```python
from build123d import *

# Parameters (mm, degrees)
F0_R     = 1.524
F1_DEPTH = 38.1
F2_R     = 25.4
F3_DEPTH = 38.101


with BuildPart() as f1:
    # F0 (on Top) → F1 (new body)
    with BuildSketch(Plane.XY):
        with BuildLine():
            ThreePointArc((30.1625, 25.4), (28.767596, 28.767596), (25.4, 30.1625))
            Line((25.4, 30.1625), (-25.4, 30.1625))
            ThreePointArc((-25.4, 30.1625), (-28.767596, 28.767596), (-30.1625, 25.4))
            Line((-30.1625, 25.4), (-30.1625, -25.4))
            ThreePointArc((-30.1625, -25.4), (-28.767596, -28.767596), (-25.4, -30.1625))
            Line((-25.4, -30.1625), (25.4, -30.1625))
            ThreePointArc((25.4, -30.1625), (28.767596, -28.767596), (30.1625, -25.4))
            Line((30.1625, -25.4), (30.1625, 25.4))
        make_face()
        with Locations((-25.4, -25.4)):
            Circle(F0_R, mode=Mode.SUBTRACT)
        with Locations((25.4, -25.4)):
            Circle(F0_R, mode=Mode.SUBTRACT)
        with Locations((-25.4, 25.4)):
            Circle(F0_R, mode=Mode.SUBTRACT)
        with Locations((25.4, 25.4)):
            Circle(F0_R, mode=Mode.SUBTRACT)
    extrude(amount=F1_DEPTH)

    # F2 (on face) → F3 (cut, through all)
    with BuildSketch(Plane.XY.offset(38.1)):
        Circle(F2_R)
    extrude(amount=-F3_DEPTH, mode=Mode.SUBTRACT)


solid = f1.part
```
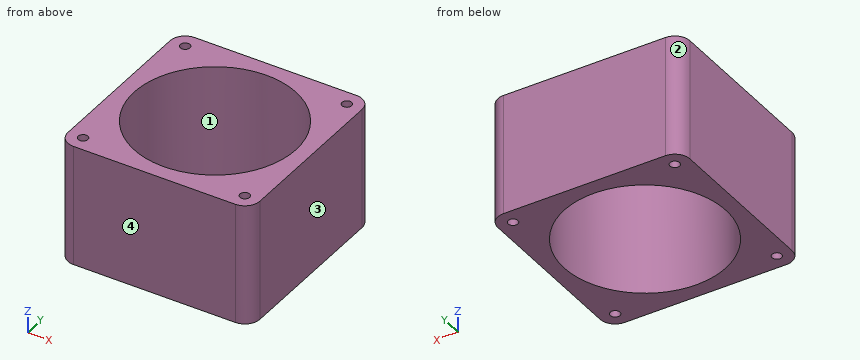
Geometry check sheet. Reference: the model listing, model coordinates, mm. Face numbers are marked on the shaded views. Coordinates: 2 decimals unless noted, no trailing zeros. Order: outer loops, then holes, each group sorted by start corner. A loop starts at its lowest first (then second) coordinate and runs counter-clockwise, first axis right, second up. Notation, with made-up numbers: M 87.25,-12 L 116.25,-12 A11 ccw 116.25,9 Z; hole C 38.25,-2.5 d10. An arc over 180 degrees is marked long. Answer as a JSON object with one key per item and string values.
Q1. Depth check by flat-ended pin: pin 1 Ø3.5 at (x, y) = (25.4, 25.4) entering from +Z. Enter the tip coordinate at first touch or a pass-through.
Results are:
{"pin 1": "stops at z = 38.1"}
Q2. Cross-section at C-C on z = 21.5. Record the cut outline in (x, y) (1 decimal), and give its area (3 significant figures).
Results are:
{"outline": "M -30.2,-25.4 A4.8 ccw -25.4,-30.2 L 25.4,-30.2 A4.8 ccw 30.2,-25.4 L 30.2,25.4 A4.8 ccw 25.4,30.2 L -25.4,30.2 A4.8 ccw -30.2,25.4 Z; hole C -25.4,-25.4 d3; hole C -25.4,25.4 d3; hole C 0,0 d50.8; hole C 25.4,-25.4 d3; hole C 25.4,25.4 d3", "area": "1,560 mm²"}
Q3. Cross-section at A-A on x = 0. Record the cut outline in (y, z), and give its area (3 significant figures).
Results are:
{"outline": "M -30.16,0 L -25.4,0 L -25.4,38.1 L -30.16,38.1 Z; M 25.4,0 L 30.16,0 L 30.16,38.1 L 25.4,38.1 Z", "area": "363 mm²"}
Q4. Cross-section at B-B on y = 9. Record the cut outline in (x, z).
Results are:
{"outline": "M -30.16,0 L -23.75,0 L -23.75,38.1 L -30.16,38.1 Z; M 23.75,0 L 30.16,0 L 30.16,38.1 L 23.75,38.1 Z"}
Q5. Release check for a two-part mould opening along Y. For the marked faces 1, 2, 3 and 4 record: released by +Y, released by -Y, zero draft, split by the parting line, or undercut.
Results are:
{"face 1": "undercut", "face 2": "released by +Y", "face 3": "zero draft", "face 4": "released by -Y"}
Q6. Scan lines: line 1 (Y direction, x = 21, z = 14); line 2 (X direction, y = 21.5, z = 31); line 3 (Y direction, x = -3, z = 35.5). Record each from-to range of solid material in increasing order.
Results are:
{"line 1": "y = -30.16 to -14.29, 14.29 to 30.16", "line 2": "x = -30.16 to -13.52, 13.52 to 30.16", "line 3": "y = -30.16 to -25.22, 25.22 to 30.16"}
